```python
from build123d import *

# Parameters (mm, degrees)
F0_W      = 101
F0_H      = 2
F1_DEPTH  = 12
F0_H_2    = 70
F2_DEPTH  = 2
F4_R      = 1.75
F5_DEPTH  = 100
F3_W      = 48
F3_H      = 12
F6_DEPTH  = 2
F7_W      = 35
F7_H      = 50
F7_W_2    = 30
F8_DEPTH  = 2
F9_W      = 5
F9_H      = 10
F10_DEPTH = 80
F11_DEPTH = 12


with BuildPart() as f1:
    # F0 (on Top) → F1 (new body)
    with BuildSketch(Plane.XY):
        Polygon((-42.3766899407, -41.0996641517), (-42.3766899407, 28.9003358483), (-42.3766899407, 30.9003358483), (-44.3766899407, 30.9003358483), (-44.3766899407, -43.0996641517), (-42.3766899407, -43.0996641517), align=None)
        with Locations((8.1233100593, 29.9003358483)):
            Rectangle(F0_W, F0_H)
        Polygon((58.6233100593, 30.9003358483), (58.6233100593, 28.9003358483), (58.6233100593, -41.0996641517), (58.6233100593, -43.0996641517), (60.6233100593, -43.0996641517), (60.6233100593, 30.9003358483), align=None)
        with Locations((8.1233100593, -42.0996641517)):
            Rectangle(F0_W, F0_H)
    extrude(amount=F1_DEPTH)

    # F0 (on Top) → F2 (join)
    with BuildSketch(Plane.XY):
        with Locations((8.1233100593, -6.0996641517)):
            Rectangle(F0_W, F0_H_2)
    extrude(amount=F2_DEPTH)

    # F4 (on face) → F5 (cut)
    with BuildSketch(Plane.XZ.offset(43.0996641517)):
        with Locations((44.6233227849, 5.0000082701)):
            Circle(F4_R)
        with Locations((-32.3766772151, 5.0000082701)):
            Circle(F4_R)
    extrude(amount=-F5_DEPTH, mode=Mode.SUBTRACT)

    # F3 (on face) → F6 (cut)
    with BuildSketch(Plane.YZ.offset(60.6233100593)):
        with Locations((-11.0996702909, 6)):
            Rectangle(F3_W, F3_H)
    extrude(amount=-F6_DEPTH, mode=Mode.SUBTRACT)

    # F7 (on face) → F8 (cut)
    with BuildSketch(Plane.XY.offset(2)):
        with Locations((-14.876691699, -6.0996547341)):
            Rectangle(F7_W, F7_H)
        with Locations((32.623308301, -6.0996547341)):
            Rectangle(F7_W_2, F7_H)
    extrude(amount=-F8_DEPTH, mode=Mode.SUBTRACT)

    # F9 (on face) → F10 (cut)
    with BuildSketch(Plane.XZ.offset(43.0996641517)):
        with Locations((-34.8767231405, 7.0000035018)):
            Rectangle(F9_W, F9_H)
        with Locations((6.1232769489, 7)):
            Rectangle(F9_W, F9_H)
        with Locations((47.1232769489, 7)):
            Rectangle(F9_W, F9_H)
    extrude(amount=-F10_DEPTH, mode=Mode.SUBTRACT)

    # F11 (cut): faces of the model
    f11_faces = [f1.faces().sort_by_distance(p)[0] for p in [
        (-14.3767230958, 29.9003358483, 12),
        (26.6232769489, 29.9003358483, 12),
        (49.8342274051, 29.9003358483, 12),
        (54.1232935041, -41.2356790884, 12),
        (26.6232769489, -42.0996641517, 12),
        (-14.3767230958, -42.0996641517, 12),
        (-42.9600276875, -6.0996641517, 12),
    ]]
    extrude(f11_faces, amount=-F11_DEPTH, mode=Mode.SUBTRACT)


solid = f1.part
```
Input: part model. Units: mm. Frame: model coordinates. A direction names the side the tool comes from. Round coordinates to 2 decimals unless told otherwise and drop trailing zeros. Loops run counter-clockwise (first coordinate to the right, second up) from the corner with the lowest first, then second, coordinate; pieces in that order, holes last. Notation, with made-up numbers: M -15,-8 L 4,-8 A22 cw 4,20 Z; hole C -30.75,22 d10. An arc over 180 degrees is marked long. Answer in a Markdown table with one row per item. Add a question column.
1. Mould query, pull axis Y, two halves, no side actions, for faces 6 (the face through (2.623, -6, 1)), 7 (the face through (-15, 28.9, 1)), 8 (the face through (47, -43.1, 1)), 9 (the face through (-35, -42, 2)). Classes: released by +Y, released by -Y, zero draft, split by the parting line, or undercut.
2. Contact query for flat-ended pins moving along their axis: pin 1 (1 mm diameter, centred on x = -40.5, z = 1, fed in from +Y); pin 2 (1 mm diameter, centred on y = 30, z = 1, fed in from -X); pin 3 (0.6 mm diameter, centred on x = -39.5, z = 1, fed in from -Y). Output: stop coordinate, or through.
3. Section A-A (x = 35). Output: boundary loops of the cut face in (y, z).
4. Ray query, probe 1 along X at (y, z) = (-23.5, 1.3); probe 2 along Y at (x, z) = (-4, 0.5); probe 3 along Y at (x, z) = (11.5, 1.25). Return the intervals inside material, ascending.
5. Section C-C (z = 0.9). Give the number of separate pieces and of enclosed holes in the cut face, and give its area (3 significant figures).
6. Set-up query: faces 1 (the face through (-40, -41.1, 1)), 2 (the face through (8.623, -42, 1)), 3 (the face through (49.623, -42, 1)), 4 (the face through (-15, 18.9, 1)), 5 (the face through (-32.377, 30, 1)). Return all of +Z, -Z, +X, -X, +Y, -Y with unobstructed straight access to the full face (end or side cutting, diameter ignored); none if empty.
7. Section B-B (y = -8). Output: boundary loops of the cut face in (x, z), and give its area (3 significant figures).
Values follow:
| question | item | result |
|---|---|---|
| 1 | face 6 | undercut |
| 1 | face 7 | released by +Y |
| 1 | face 8 | released by -Y |
| 1 | face 9 | zero draft |
| 2 | pin 1 | y = 28.9 |
| 2 | pin 2 | x = -37.38 |
| 2 | pin 3 | y = -41.1 |
| 3 | outline | M -41.1,0 L -31.1,0 L -31.1,2 L -41.1,2 Z; M 18.9,0 L 28.9,0 L 28.9,2 L 18.9,2 Z |
| 4 | probe 1 | -42.38 to -32.38, 2.62 to 17.62, 47.62 to 58.62 |
| 4 | probe 2 | -41.1 to -31.1, 18.9 to 28.9 |
| 4 | probe 3 | -41.1 to 28.9 |
| 5 | separate pieces | 1 |
| 5 | enclosed holes | 2 |
| 5 | area | 3,880 mm^2 |
| 6 | face 1 | +Z, -Z, -X, -Y |
| 6 | face 2 | +Z, -Z, -Y |
| 6 | face 3 | +Z, -Z, +X, -Y |
| 6 | face 4 | +Z, -Z |
| 6 | face 5 | +Z, -Z, +Y |
| 7 | outline | M -42.38,0 L -32.38,0 L -32.38,2 L -42.38,2 Z; M 2.62,0 L 17.62,0 L 17.62,2 L 2.62,2 Z; M 47.62,0 L 58.62,0 L 58.62,2 L 47.62,2 Z |
| 7 | area | 72.0 mm^2 |
